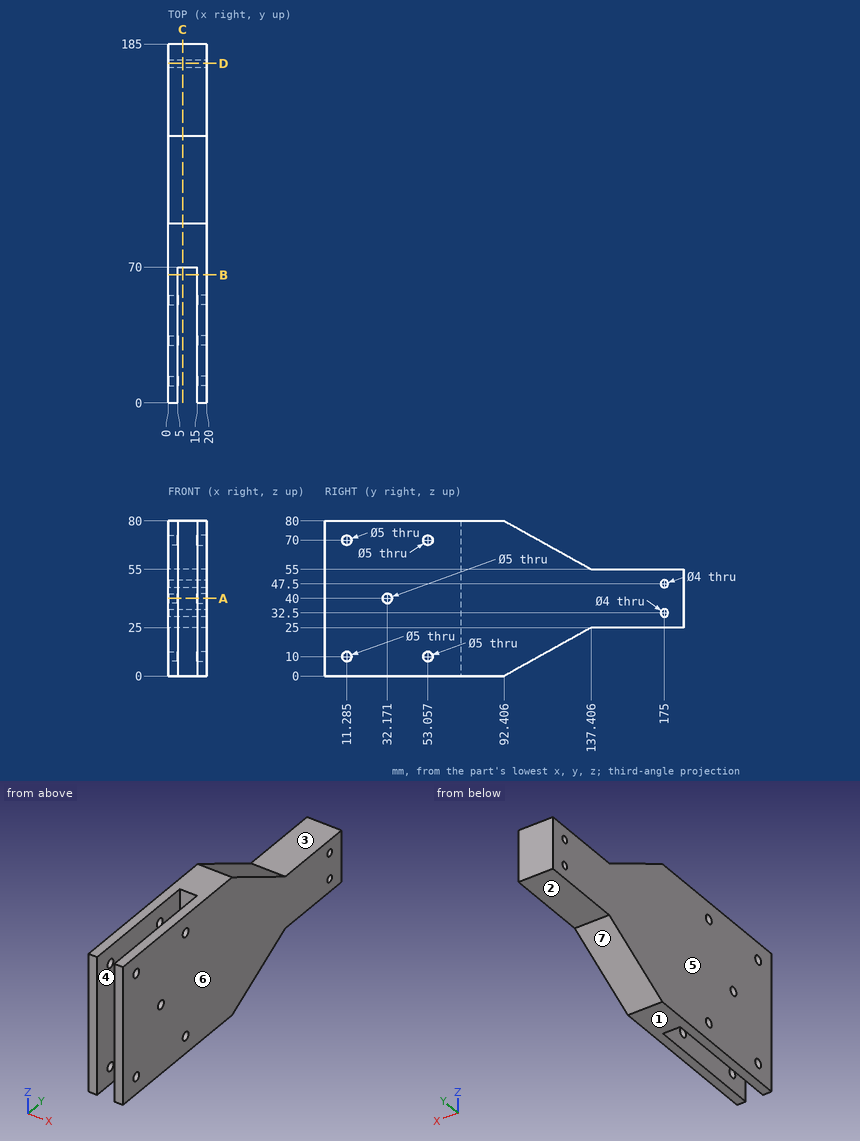
Input: dimensioned drawing with shaded views. Units: mm. Origin: part minimum x, y, z. A direction names the side the tool comes from. Give positions to 0.01 mm unless a question says otherwise; leave off trailing zeros. Write each loop counter-clockwise with the first axis right and the second up, starting at its lowest first coordinate (ties: lowest second). Pieces come first, ordered by that corner, then holes. Notation, with made-up numbers: (-10.75, -18.75) -> (10.25, -18.75) arc R29 ccw to (10.25, 20.25) -> close; hole circle Ø6 at (6, 74). An arc over 180 degrees is marked (long way). Return JSON: item names as keys, results as strings. Group by question number.
1. Access query for the marked faces 1, 2 and 3. Directions: +Z, -Z, +X, -X, +Y, -Y. A direction counts if a zero-diameter tool reaches every point of the face in a straight line with its end or side. Return the directions, or none.
2. Section D-D, the plane y = 175. Output: boundary loops of the cut face in (x, z).
3. Section C-C, the plane x = 7.5. Output: boundary loops of the cut face in (y, z), then the cut area to 3 significant figures.
4. Mould query, pull axis X, two halves, no side actions, for the marked faces 4, 5, 6 and 7. Classes: +X half, -X half, draft (parallel to the pull), parting line (faces both ways), or undercut.
5. Material intervals for line 1 (Z direction, x = 11.25, y = 175); line 2 (X direction, y = 27, z = 44); line 3 (Y direction, x = 16, z = 10) (1 decimal), sorted ascending. Write a range as from..to.
6. Section A-A, the plane z = 40. Output: boundary loops of the cut face in (x, y), then the cut area to 3 significant figures.
7. Section B-B, the plane y = 66. Output: boundary loops of the cut face in (x, z).
8. Pin query (flat end, axial travel): pin 1 Ø10 at (y, z) = (34, 24) entering from -X; pin 2 Ø12 at (x, z) = (9, 64) entering from +Y (1 decimal); pin 3 Ø10 at (x, y) = (5.5, 155) entering from +Z; pin 4 Ø8 at (x, y) = (7, 116) entering from -Z (1 decimal). Return the tip coordinate at first contact, or that it passes through.
Determined:
{
 "1": {"face 1": "-Z, +X, -X, +Y, -Y", "face 2": "-Z, +X, -X, +Y", "face 3": "+Z, +X, -X, +Y"},
 "2": {"outline": "(0, 25) -> (20, 25) -> (20, 30.5) -> (0, 30.5) -> close; (0, 34.5) -> (20, 34.5) -> (20, 45.5) -> (0, 45.5) -> close; (0, 49.5) -> (20, 49.5) -> (20, 55) -> (0, 55) -> close"},
 "3": {"outline": "(70, 0) -> (92.41, 0) -> (137.41, 25) -> (185, 25) -> (185, 55) -> (137.41, 55) -> (92.41, 80) -> (70, 80) -> close; hole circle Ø4 at (175, 32.5); hole circle Ø4 at (175, 47.5)", "area": "5,670 mm2"},
 "4": {"face 4": "undercut", "face 5": "-X half", "face 6": "+X half", "face 7": "draft"},
 "5": {"line 1": "z = 25..30.5, 34.5..45.5, 49.5..55", "line 2": "x = 0..5, 15..20", "line 3": "y = 0..8.8, 13.8..50.6, 55.6..110.4"},
 "6": {"outline": "(0, 0) -> (5, 0) -> (5, 29.67) -> (0, 29.67) -> close; (0, 34.67) -> (5, 34.67) -> (5, 70) -> (15, 70) -> (15, 34.67) -> (20, 34.67) -> (20, 185) -> (0, 185) -> close; (15, 0) -> (20, 0) -> (20, 29.67) -> (15, 29.67) -> close", "area": "2,950 mm2"},
 "7": {"outline": "(0, 0) -> (5, 0) -> (5, 80) -> (0, 80) -> close; (15, 0) -> (20, 0) -> (20, 80) -> (15, 80) -> close"},
 "8": {"pin 1": "stops at x = 0", "pin 2": "stops at y = 132", "pin 3": "stops at z = 55", "pin 4": "stops at z = 10.9"}
}
